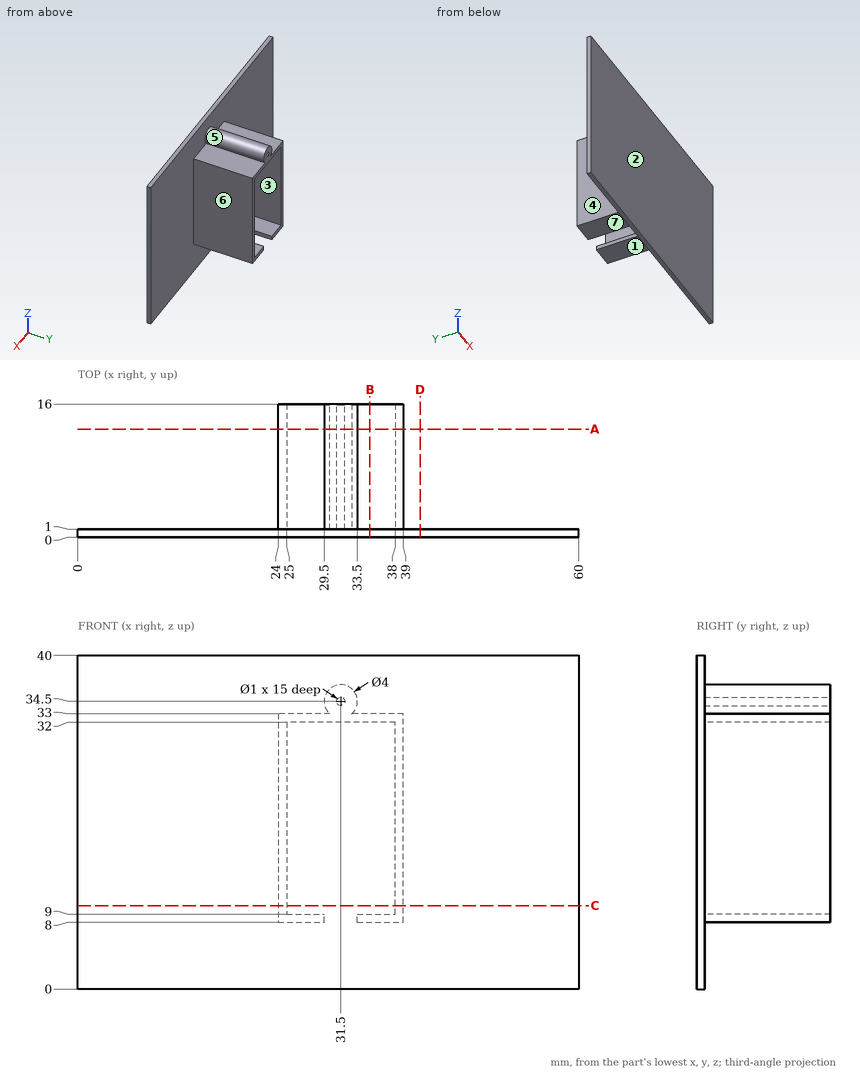
For this review, use the dimensioned drawing (mm, ordinates from the lowest corner) and the shaded views. A direction names the side the tool comes from. Round coordinates to 2 decimals unless told otherwise and drop trailing zeros. Write each loop counter-clockwise with the first axis right and the second up, starting at its lowest first coordinate (ties: lowest second). Pieces come first, ordered by that corner, then holes. Notation, with made-up numbers: M 37.25,48 L 87.25,48 A20 ccw 87.25,80 Z; hole C -40,-23 d3. An arc over 180 degrees is marked long. Answer as CSV lines item,"result". Start each with the question number.
Q1. Consider section C-C, the plane z = 10. Give the boundary of the cut face in (x, y), then the cut area to 3 significant figures.
Q2. The part is to be moulded in two halves that separate along Z. For the marked faces 5, 6 and 7, say which applies: +Z half, -Z half, draft (parallel to the pull), parting line (faces both ways), or undercut.
Q3. Consider section D-D, the plane x = 41. Give the boundary of the cut face in (y, z).
Q4. Clearance check with flat-ended pins moving along their axes: P1, Ø5, axis at y = 14, z = 18.5, coming from the -X side; P2, Ø1.6, axis at x = 36.5, y = 6.5, coming from the -Z side; P3, Ø0.8, axis at y = 5.5, z = 8.5, coming from the +X side; P4, Ø6, axis at x = 18.5, y = 9.5, coming from the +Z side. State where each tip first meets the part, or that it passes through.
Q5. Tool access review of the marked faces 1, 2, 3 and 4: name each direction out of +Z, -Z, +X, -X, +Y, -Y from which nothing blocks a thin tool from reaching the whole face with its end or side.
Q6. Consider section A-A, the plane y = 13. Give the boundary of the cut face in (x, z).
Q7. Wall thickness on line 1 along X through (y, z) = (11, 34.5); line 2 along Z through (x, y) = (31.5, 4.75); line 3 along X through (y, z) = (5.25, 19): over which ranges is each line inside the solid? List them lowest first.
Q8. Consider section B-B, the plane x = 35. Give the boundary of the cut face in (y, z).
Result set:
1,outline,"M 0,0 L 60,0 L 60,1 L 39,1 L 39,16 L 38,16 L 38,1 L 25,1 L 25,16 L 24,16 L 24,1 L 0,1 Z"
1,area,"90.0 mm²"
2,face 5,"undercut"
2,face 6,"draft"
2,face 7,"-Z half"
3,outline,"M 0,0 L 1,0 L 1,40 L 0,40 Z"
4,P1,"stops at x = 24"
4,P2,"stops at z = 8"
4,P3,"stops at x = 39"
4,P4,"passes through"
5,face 1,"-Z, +X, -X, +Y"
5,face 2,"+Z, -Z, +X, -X, -Y"
5,face 3,"+Y"
5,face 4,"+Z, -Z, -X, +Y"
6,outline,"M 24,8 L 29.5,8 L 29.5,9 L 25,9 L 25,32 L 38,32 L 38,9 L 33.5,9 L 33.5,8 L 39,8 L 39,33 L 32.82,33 A2 ccw long 30.18,33 L 24,33 Z; hole C 31.5,34.5 d1"
7,line 1,"x = 29.5 to 31, 32 to 33.5"
7,line 2,"z = 32 to 34, 35 to 36.5"
7,line 3,"x = 24 to 25, 38 to 39"
8,outline,"M 0,0 L 1,0 L 1,8 L 16,8 L 16,9 L 1,9 L 1,32 L 16,32 L 16,33 L 1,33 L 1,40 L 0,40 Z"
